Source: CAD feature listing. Evaluate the final solid. Frame: model axes, mm. Face numbers are marked on the shaded views. A direction names the side the tool comes from. Give positions to 0.01 mm unless a question says otherwise; leave off trailing zeros. Loops run counter-clockwise (first coordinate to the right, second up) from the corner with the lowest first, then second, coordinate; pieces in that order, holes last. Notation, with made-up numbers: M 72,71 L 113,71 A26 cw 113,93 Z; hole C 58.25,2 d5. An arc over 180 degrees is marked long. Answer in a Markdown table with one row per item.
```python
from build123d import *

# Parameters (mm, degrees)
BOSS_EXTRUDE1_START = -12.5
BOSS_EXTRUDE1_DEPTH = 6.5
SKETCH1_3_R         = 6
BOSS_EXTRUDE2_DEPTH = 12.5


with BuildPart() as part:
    # Sketch1 → Boss-Extrude1 (new body)
    with BuildSketch(Plane.XY.offset(BOSS_EXTRUDE1_START)):
        with BuildLine():
            Line((0, 95), (43.964466094, 51.035533906))
            ThreePointArc((43.964466094, 51.035533906), (45.428932188, 47.5), (43.964466094, 43.964466094))
            Line((43.964466094, 43.964466094), (0, 0))
            Line((0, 0), (100, 0))
            Line((100, 0), (52.5, 47.5))
            Line((52.5, 47.5), (100, 95))
            Line((100, 95), (0, 95))
        make_face()
    boss_extrude1 = extrude(amount=BOSS_EXTRUDE1_DEPTH)

    # Sketch1_3 → Boss-Extrude2 (add, symmetric)
    with BuildSketch(Plane.XY):
        with BuildLine():
            ThreePointArc((43.964466094, 51.035533906), (45.428932188, 47.5), (43.964466094, 43.964466094))
            Line((43.964466094, 43.964466094), (0, 0))
            Line((0, 0), (0, 95))
            Line((0, 95), (43.964466094, 51.035533906))
        make_face()
        with Locations((20, 47.5)):
            Circle(SKETCH1_3_R, mode=Mode.SUBTRACT)
    extrude(amount=BOSS_EXTRUDE2_DEPTH, both=True)

    # Mirror2: Boss-Extrude1 across plane
    add(boss_extrude1.mirror(Plane.XY))


solid = part.part
```
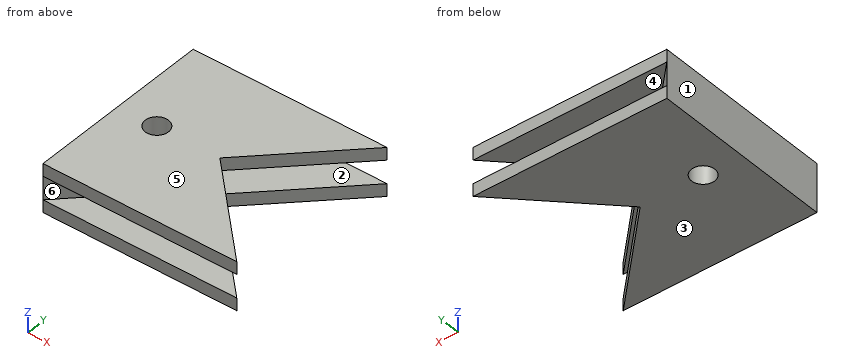
1) Pull-direction query (Z, two-part tool) for the marked faces 1, 2 and 3; classes: released by +Z, released by -Z, zero draft, split by the parting line, or undercut.
Reply:
| item | result |
|---|---|
| face 1 | zero draft |
| face 2 | undercut |
| face 3 | released by -Z |
2) Pin query (flat end, axial travel): pin 1 Ø8 at (y, z) = (43.5, 0.5) entering from +X; pin 2 Ø10 at (x, z) = (19.5, 0.5) entering from +Y; pin 3 Ø9.5 at (x, y) = (20, 47.5) entering from -Z. Return the tip coordinate at first contact, or that it passes through.
Reply:
| item | result |
|---|---|
| pin 1 | stops at x = 45.43 |
| pin 2 | stops at y = 80.5 |
| pin 3 | passes through |
3) Material intervals for L1, parallel to Z at x = 33, y = 85; L2, parallel to Y at x = 20, z = 7.5; L3, parallel to Y at x = 23.5, z = 11.25, sorted ascending.
Reply:
| item | result |
|---|---|
| L1 | z = -12.5 to -6, 6 to 12.5 |
| L2 | y = 0 to 41.5, 53.5 to 95 |
| L3 | y = 0 to 42.63, 52.37 to 95 |
4) Section D-D, the plane y = 88. Return loops of the section in (x, z).
Reply:
| item | result |
|---|---|
| outline | M 0,-12.5 L 93,-12.5 L 93,-6 L 7,-6 L 7,6 L 93,6 L 93,12.5 L 0,12.5 Z |
5) Section B-B, the plane x = 48.5. Return loops of the section in (y, z).
Reply:
| item | result |
|---|---|
| outline | M 0,-12.5 L 95,-12.5 L 95,-6 L 0,-6 Z; M 0,6 L 95,6 L 95,12.5 L 0,12.5 Z |
6) Set-up query: the marked faces 4, 5 and 6. Return all of +Z, -Z, +X, -X, +Y, -Y with unobstructed straight access to the full face (end or side cutting, diameter ignored); none if empty.
Reply:
| item | result |
|---|---|
| face 4 | +X |
| face 5 | +Z, +X, -X, +Y, -Y |
| face 6 | +X, -Y |
7) Section A-A, the plane x = 78.5. Return loops of the section in (y, z).
Reply:
| item | result |
|---|---|
| outline | M 0,-12.5 L 21.5,-12.5 L 21.5,-6 L 0,-6 Z; M 0,6 L 21.5,6 L 21.5,12.5 L 0,12.5 Z; M 73.5,-12.5 L 95,-12.5 L 95,-6 L 73.5,-6 Z; M 73.5,6 L 95,6 L 95,12.5 L 73.5,12.5 Z |
8) Section C-C, the plane z = 9.25. Return loops of the section in (x, y).
Reply:
| item | result |
|---|---|
| outline | M 0,0 L 100,0 L 52.5,47.5 L 100,95 L 0,95 Z; hole C 20,47.5 d12 |
